Could you check a few things on this drawing? It's one solid part, dimensions in mm from its lowest x, y, z. Give positions to 0.01 mm unless a question says otherwise; leave off trailing zeros. Loops run counter-clockwise (first coordinate to the right, second up) from the corner with the lowest first, then second, coordinate; pieces in that order, holes last.
1. Imagine slicing it at C-C (y = 2.35). List the corners of the cut face in (x, z) for me, plus the area to 3 significant figures.
2. Imagine slicing it at D-D (z = 21). List the corners of the cut face in (x, y) for me.
3. For P1, Ø10, axis at x = 9, z = 21.5, coming from the +Y side, with a flat end and sliding along its axis, tell me the tip position at first contact or that it passes through.
4. I need wall thicknesses on line 1 along Z through (x, y) = (6, 2.3); line 2 along X through (y, z) = (1.05, 2.3); line 3 along X through (y, z) = (1.75, 22). Which ranges of each line are inside material? Lowest first, please.
5. Imagine slicing it at A-A (x = 10.5). List the corners of the cut face in (y, z) for me.
6. Imagine slicing it at B-B (z = 29.6). List the corners of the cut face in (x, y) for me.
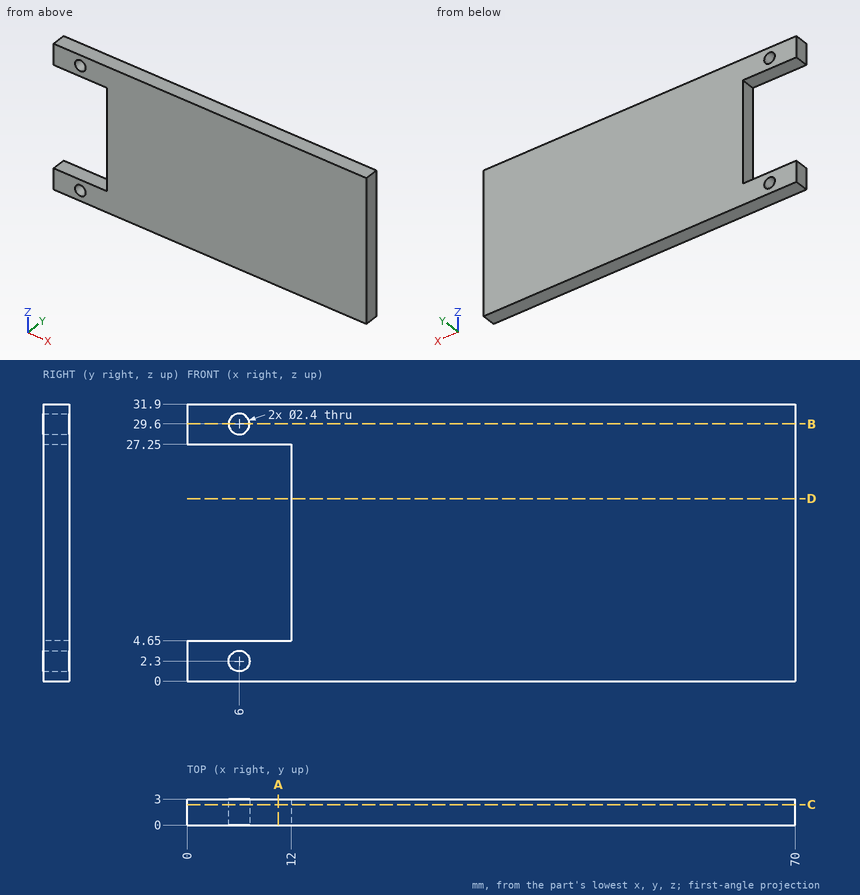
Derived:
1. outline: (0, 0) - (70, 0) - (70, 31.9) - (0, 31.9) - (0, 27.25) - (12, 27.25) - (12, 4.65) - (0, 4.65) - close; hole circle Ø2.4 at (6, 2.3); hole circle Ø2.4 at (6, 29.6)
1. area: 1,950 mm2
2. outline: (12, 0) - (70, 0) - (70, 3) - (12, 3) - close
3. P1: stops at y = 3
4. line 1: z = 0 to 1.1, 3.5 to 4.65, 27.25 to 28.4, 30.8 to 31.9
4. line 2: x = 0 to 4.8, 7.2 to 70
4. line 3: x = 12 to 70
5. outline: (0, 0) - (3, 0) - (3, 4.65) - (0, 4.65) - close; (0, 27.25) - (3, 27.25) - (3, 31.9) - (0, 31.9) - close
6. outline: (0, 0) - (4.8, 0) - (4.8, 3) - (0, 3) - close; (7.2, 0) - (70, 0) - (70, 3) - (7.2, 3) - close
